Part model, mm, in its own coordinate system. Face numbers are marked on the shaded views. A direction names the side the tool comes from. Coordinates: 2 decimals unless noted, no trailing zeros. Order: outer loops, then holes, each group sorted by start corner. A loop starts at its lowest first (then second) coordinate and runs counter-clockwise, first axis right, second up. Notation, with made-up numbers: (-23, 14.5) - (-9, 14.5) arc R27 ccw to (-9, 33.5) - close; hole circle Ø7 at (-1, 31.5). An arc over 180 degrees is marked (long way). Use a Markdown table: item, result. Add a question column.
1) Saw through at B-B on x = 25.5. List the corners of the cut face in (y, z), then the cut area to 3 significant figures.
2) Saw through at A-A on z = -10.5. List the corners of the cut face in (x, y), then the cut area to 3 significant figures.
3) Drop flat-ended pins along their axis: P1, Ø17, axis at y = 18.5, z = -2.5, coming from the -X side; P2, Ø10, axis at y = 4, z = -3, coming from the +X side; P3, Ø1.5, axis at x = 25.5, z = 10.5, coming from the +Y side; P4, Ø1.5, axis at x = 33.5, z = -12.5, coming from the -Y side. Give the stop position or say it passes through.
4) Saw through at C-C on z = 13. List the corners of the cut face in (x, y), then the cut area to 3 significant figures.
5) Saw through at D-D on y = 13.5. List the corners of the cut face in (x, z), then the cut area to 3 significant figures.
6) Tool access for the marked faces 1, 2 and 3: list every direction of +Z, -Z, +X, -X, +Y, -Y with a clear straight run to the whole face (end or side of a thin tool).
7) Wall check: L1, parallel to X at y = 2.25, z = 13; L2, parallel to X at y = 27.85, z = -10.5; L3, parallel to X at y = 19.5, z = 0.5. Give the ranges that are in metal, low to high. Write a range as [from, to].
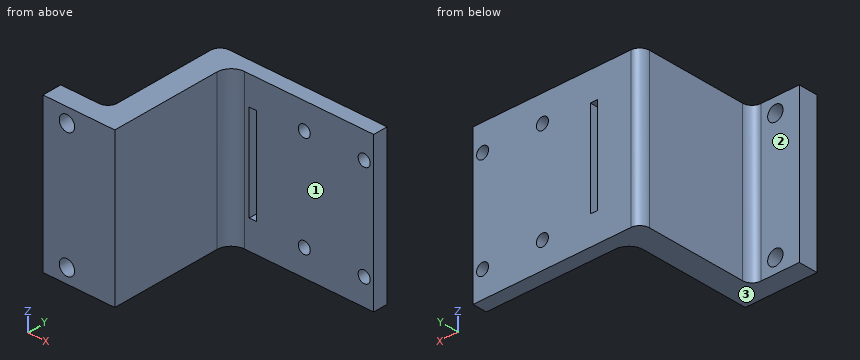
```python
from build123d import *

# Parameters (mm, degrees)
SKETCH1_W           = 10
SKETCH1_H           = 32
SKETCH1_R           = 1.6
BOSS_EXTRUDE1_DEPTH = 4
SKETCH2_W           = 32
SKETCH2_H           = 4
BOSS_EXTRUDE2_DEPTH = 5
SKETCH3_W           = 5
SKETCH3_H           = 32
BOSS_EXTRUDE3_DEPTH = 25
FILLET1_R           = 2
SKETCH4_W           = 32
SKETCH4_H           = 3
BOSS_EXTRUDE4_DEPTH = 30
SKETCH5_R           = 1.25
CUT_EXTRUDE1_DEPTH  = 25
FILLET2_R           = 2
FILLET3_R           = 3
SKETCH7_W           = 1.5
SKETCH7_H           = 20
CUT_EXTRUDE2_DEPTH  = 10


with BuildPart() as part:
    # Sketch1 → Boss-Extrude1 (new body)
    with BuildSketch(Plane(origin=(0, 0, 0), x_dir=(1, 0, 0), z_dir=(0, 1, 0))):
        Rectangle(SKETCH1_W, SKETCH1_H)
        with Locations(Location((0, -13, 0), (0, 0, 270))):
            Circle(SKETCH1_R, mode=Mode.SUBTRACT)
        with Locations(Location((0, 13, 0), (0, 0, 270))):
            Circle(SKETCH1_R, mode=Mode.SUBTRACT)
    extrude(amount=BOSS_EXTRUDE1_DEPTH)

    # Sketch2 → Boss-Extrude2 (add)
    with BuildSketch(Plane(origin=(5, 0, 0), x_dir=(0, 0, -1), z_dir=(1, 0, 0))):
        with Locations((0, 2)):
            Rectangle(SKETCH2_W, SKETCH2_H)
    extrude(amount=BOSS_EXTRUDE2_DEPTH)

    # Sketch3 → Boss-Extrude3 (add)
    with BuildSketch(Plane(origin=(0, 4, 0), x_dir=(1, 0, 0), z_dir=(0, 1, 0))):
        with Locations((7.5, 0)):
            Rectangle(SKETCH3_W, SKETCH3_H)
    extrude(amount=BOSS_EXTRUDE3_DEPTH)

    # Fillet1
    fillet1_edges = [part.edges().sort_by_distance(p)[0] for p in [
        (5, 4, 0),
    ]]
    fillet(fillet1_edges, radius=FILLET1_R)

    # Sketch4 → Boss-Extrude4 (add)
    with BuildSketch(Plane(origin=(10, 0, 0), x_dir=(0, 0, -1), z_dir=(1, 0, 0))):
        with Locations((0, 27.5)):
            Rectangle(SKETCH4_W, SKETCH4_H)
    extrude(amount=BOSS_EXTRUDE4_DEPTH)

    # Sketch5 → Cut-Extrude1 (cut)
    with BuildSketch(Plane(origin=(0, 29, 0), x_dir=(1, 0, 0), z_dir=(0, 1, 0))):
        with Locations(Location((38, -10.5, 0), (0, 0, 270))):
            Circle(SKETCH5_R)
        with Locations(Location((38, 10.5, 0), (0, 0, 270))):
            Circle(SKETCH5_R)
        with Locations(Location((25.5, 10.5, 0), (0, 0, 270))):
            Circle(SKETCH5_R)
        with Locations(Location((25.5, -10.5, 0), (0, 0, 270))):
            Circle(SKETCH5_R)
    extrude(amount=-CUT_EXTRUDE1_DEPTH, mode=Mode.SUBTRACT)

    # Fillet2
    fillet2_edges = [part.edges().sort_by_distance(p)[0] for p in [
        (5, 29, 0),
    ]]
    fillet(fillet2_edges, radius=FILLET2_R)

    # Fillet3
    fillet3_edges = [part.edges().sort_by_distance(p)[0] for p in [
        (10, 26, 0),
    ]]
    fillet(fillet3_edges, radius=FILLET3_R)

    # Sketch7 → Cut-Extrude2 (cut)
    with BuildSketch(Plane.XZ.offset(-26)):
        with Locations((14.75, 0)):
            Rectangle(SKETCH7_W, SKETCH7_H)
    extrude(amount=-CUT_EXTRUDE2_DEPTH, mode=Mode.SUBTRACT)


solid = part.part
```
Results are:
| question | item | result |
|---|---|---|
| 1 | outline | (26, -16) - (29, -16) - (29, -11.75) - (26, -11.75) - close; (26, -9.25) - (29, -9.25) - (29, 9.25) - (26, 9.25) - close; (26, 11.75) - (29, 11.75) - (29, 16) - (26, 16) - close |
| 1 | area | 81.0 mm2 |
| 2 | outline | (-5, 0) - (10, 0) - (10, 23) arc R3 cw to (13, 26) - (24.25, 26) - (24.25, 29) - (7, 29) arc R2 ccw to (5, 27) - (5, 6) arc R2 cw to (3, 4) - (-5, 4) - close; (26.75, 26) - (36.75, 26) - (36.75, 29) - (26.75, 29) - close; (39.25, 26) - (40, 26) - (40, 29) - (39.25, 29) - close |
| 2 | area | 262 mm2 |
| 3 | P1 | x = 5 |
| 3 | P2 | x = 10 |
| 3 | P3 | through |
| 3 | P4 | y = 26 |
| 4 | outline | (-5, 0) - (-1.6, 0) - (-1.6, 4) - (-5, 4) - close; (1.6, 0) - (10, 0) - (10, 23) arc R3 cw to (13, 26) - (40, 26) - (40, 29) - (7, 29) arc R2 ccw to (5, 27) - (5, 6) arc R2 cw to (3, 4) - (1.6, 4) - close |
| 4 | area | 264 mm2 |
| 5 | outline | (5, -16) - (10, -16) - (10, 16) - (5, 16) - close |
| 5 | area | 160 mm2 |
| 6 | face 1 | +Z, -Z, +X, -Y |
| 6 | face 2 | +Z, -Z, -X, +Y |
| 6 | face 3 | -Z, +X, -X, +Y, -Y |
| 7 | L1 | [-5, -1.6], [1.6, 10] |
| 7 | L2 | [5.19, 24.25], [26.75, 36.75], [39.25, 40] |
| 7 | L3 | [5, 10] |
